The listing builds one solid part. Answer for the finished solid, in the listing's coordinates (mm). A direction names the side the tool comes from. Round coordinates to 2 decimals unless told otherwise and drop trailing zeros. Loops run counter-clockwise (first coordinate to the right, second up) from the corner with the lowest first, then second, coordinate; pieces in that order, holes last. Notation, with made-up numbers: (53.5, -17) -> (102.5, -17) arc R17 ccw to (102.5, 3) -> close; hole circle Ø3 at (67, 32.25). An arc over 180 degrees is marked (long way). Use a Markdown table: item, result. Add a question column.
Q1. For a pull along Y with two mould halves and no side action, classify faces 1 (the cylindrical face through (103.746, -24.724, 1.282)), 2 (the cylindrical face through (-3.57, -28.9, 1.31)), 3 (the cylindrical face through (-4, 3, 1)) as released by +Y, released by -Y, zero draft, split by the parting line, or undercut.
Q2. Section B-B on y = -20 is taken. Give the vertices of the cut face in (x, z).
Q3. Section D-D on x = 64.5 is taken. Give the vertices of the cut face in (y, z).
Q4. Which of the six approach directions +Z, -Z, +X, -X, +Y, -Y give full straight-line access (tool end or side, diameter ignored) to faces 4 (the cylindrical face through (-0.29, -23.17, 1.28)), 5 (the cylindrical face through (95.1, -6.43, 1.31))?
Q5. Section C-C on z = 1.2 is taken. Give the number of separate pieces and of enclosed holes in the cut face, then the cut area to 3 significant figures.
Q6. Given pin 1 Ø3.5 at (x, y) = (0, 0) entering from -Z, flat-ended and moving along its own axis, determine where the tip first touches the part or whether it passes through.
Q7. Consider line 1 (Y direction, x = 0, z = 0.8); line 2 (X direction, y = -17, z = 1.7); line 3 (X direction, y = -27, z = 1.55). Determine where each line is inside the solid, lowest interval first.
Q8. Section A-A on x = 50.8 is taken. Give the vertices of the cut face in (y, z).
from build123d import *

# Parameters (mm, degrees)
SKETCH1_R           = 2.25
BOSS_EXTRUDE1_DEPTH = 2.6
FILLET1_R           = 5
FILLET2_R           = 0.5


with BuildPart() as part:
    # Sketch1 → Boss-Extrude1 (new body)
    with BuildSketch(Plane.XY):
        Polygon((-5, 5), (-5, -30.4), (5, -30.4), (5, -5), (96.6, -5), (96.6, -30.4), (106.6, -30.4), (106.6, 5), align=None)
        Circle(SKETCH1_R, mode=Mode.SUBTRACT)
        with Locations((101.6, 0)):
            Circle(SKETCH1_R, mode=Mode.SUBTRACT)
        with Locations((0, -25.4)):
            Circle(SKETCH1_R, mode=Mode.SUBTRACT)
        with Locations((101.6, -25.4)):
            Circle(SKETCH1_R, mode=Mode.SUBTRACT)
        with Locations((50.8, 0)):
            Circle(SKETCH1_R, mode=Mode.SUBTRACT)
    extrude(amount=BOSS_EXTRUDE1_DEPTH)

    # Fillet1
    fillet1_edges = [part.edges().sort_by_distance(p)[0] for p in [
        (96.6, -30.4, 1.3),
        (106.6, -30.4, 1.3),
        (106.6, 5, 1.3),
        (96.6, -5, 1.3),
        (-5, 5, 1.3),
        (-5, -30.4, 1.3),
        (5, -30.4, 1.3),
        (5, -5, 1.3),
    ]]
    fillet(fillet1_edges, radius=FILLET1_R - 0.0001)  # a hair under: the kernel refuses the full size

    # Fillet2
    fillet2_edges = [part.edges().sort_by_distance(p)[0] for p in [
        (96.6, -17.7, 0),
        (50.8, -5, 0),
        (5, -17.7, 0),
        (-5, -12.7, 0),
        (50.8, 5, 0),
        (106.6, -12.7, 0),
        (3.535563195, -28.935563195, 0),
        (-3.535563195, -28.935563195, 0),
        (-3.535563195, 3.535563195, 0),
        (105.135563195, 3.535563195, 0),
        (105.135563195, -28.935563195, 0),
        (98.064436805, -28.935563195, 0),
        (96.6, -17.7, 2.6),
        (106.6, -12.7, 2.6),
        (50.8, 5, 2.6),
        (-5, -12.7, 2.6),
        (5, -17.7, 2.6),
        (50.8, -5, 2.6),
        (3.535563195, -28.935563195, 2.6),
        (-3.535563195, -28.935563195, 2.6),
        (-3.535563195, 3.535563195, 2.6),
        (105.135563195, 3.535563195, 2.6),
        (105.135563195, -28.935563195, 2.6),
        (98.064436805, -28.935563195, 2.6),
        (95.135563195, -6.464436805, 0),
        (95.135563195, -6.464436805, 2.6),
        (6.464436805, -6.464436805, 0),
        (6.464436805, -6.464436805, 2.6),
    ]]
    fillet(fillet2_edges, radius=FILLET2_R)


solid = part.part
Checked values:
| question | item | result |
|---|---|---|
| 1 | face 1 | undercut |
| 1 | face 2 | released by -Y |
| 1 | face 3 | released by +Y |
| 2 | outline | (-5, 0.5) arc R0.5 ccw to (-4.5, 0) -> (4.5, 0) arc R0.5 ccw to (5, 0.5) -> (5, 2.1) arc R0.5 ccw to (4.5, 2.6) -> (-4.5, 2.6) arc R0.5 ccw to (-5, 2.1) -> close; (96.6, 0.5) arc R0.5 ccw to (97.1, 0) -> (106.1, 0) arc R0.5 ccw to (106.6, 0.5) -> (106.6, 2.1) arc R0.5 ccw to (106.1, 2.6) -> (97.1, 2.6) arc R0.5 ccw to (96.6, 2.1) -> close |
| 3 | outline | (-5, 0.5) arc R0.5 ccw to (-4.5, 0) -> (4.5, 0) arc R0.5 ccw to (5, 0.5) -> (5, 2.1) arc R0.5 ccw to (4.5, 2.6) -> (-4.5, 2.6) arc R0.5 ccw to (-5, 2.1) -> close |
| 4 | face 4 | +Z, -Z |
| 4 | face 5 | +Z, -Z, -Y |
| 5 | separate pieces | 1 |
| 5 | enclosed holes | 5 |
| 5 | area | 1,520 mm2 |
| 6 | pin 1 | passes through |
| 7 | line 1 | y = -30.4 to -27.65, -23.15 to -2.25, 2.25 to 5 |
| 7 | line 2 | x = -5 to 5, 96.6 to 106.6 |
| 7 | line 3 | x = -4.74 to -1.58, 1.58 to 4.74, 96.86 to 100.02, 103.18 to 106.34 |
| 8 | outline | (-5, 0.5) arc R0.5 ccw to (-4.5, 0) -> (-2.25, 0) -> (-2.25, 2.6) -> (-4.5, 2.6) arc R0.5 ccw to (-5, 2.1) -> close; (2.25, 0) -> (4.5, 0) arc R0.5 ccw to (5, 0.5) -> (5, 2.1) arc R0.5 ccw to (4.5, 2.6) -> (2.25, 2.6) -> close |
